Design review of the part built by this model. Coordinates are the model's own, in mm. A direction names the side the tool comes from. Round coordinates to 2 decimals unless told otherwise and drop trailing zeros. Order: outer loops, then holes, each group sorted by start corner. A loop starts at its lowest first (then second) coordinate and runs counter-clockwise, first axis right, second up.
from build123d import *

# Parameters (mm, degrees)
F0_R     = 5.55625
F1_DEPTH = 4.7625
F2_R     = 2.2225
F3_DEPTH = 12.7
F4_R     = 1.5875
F5_DEPTH = 11.5443


# Not quite as in the source:
# - a length typed as a fraction of an inch, garbled in the dataset ("3 / 203.2 mm" for 3/8 in), is restored


with BuildPart() as f1:
    # F0 (on Top) → F1 (new body)
    with BuildSketch(Plane.XY):
        Circle(F0_R)
    extrude(amount=F1_DEPTH)

    # F2 (on face) → F3 (join)
    with BuildSketch(Plane.XY.offset(4.7625)):
        Circle(F2_R)
    extrude(amount=F3_DEPTH)

    # F4 (on face) → F5 (join)
    with BuildSketch(Plane(origin=(0, 0, 0), x_dir=(1, 0, 0), z_dir=(0, 0, -1))):
        Circle(F4_R)
    extrude(amount=F5_DEPTH)


solid = f1.part
1) Take a section at C-C on z = 13.25. Give the boundary of the cut face in (x, y) (1 decimal).
Results:
outline: circle Ø4.4 at (0, 0)
2) For faces 1 (the face through (-0.1, -2.4, 4.762)), 2 (the face through (5.3, 1.67, 2.35)), 3 (the face through (-1.3, -1.2, 0)), list the 3-axis set-ups (+Z, -Z, +X, -X, +Y, -Y) from which the entire face can be reached by the end or side of a thin tool; tool diameter is ignored.
Results:
face 1: +Z
face 2: +Z, -Z
face 3: -Z
3) Take a section at A-A on x = 0. Give the boundary of the cut face in (y, z), plus the area to 3 significant figures.
Results:
outline: (-5.56, 0) - (-1.59, 0) - (-1.59, -11.54) - (1.59, -11.54) - (1.59, 0) - (5.56, 0) - (5.56, 4.76) - (2.22, 4.76) - (2.22, 17.46) - (-2.22, 17.46) - (-2.22, 4.76) - (-5.56, 4.76) - close
area: 146 mm2
4) Take a section at D-D on x = 2.5. Give the boundary of the cut face in (y, z).
Results:
outline: (-4.96, 0) - (4.96, 0) - (4.96, 4.76) - (-4.96, 4.76) - close
5) Clearance check with flat-ended pins moving along their axes: P1, Ø4, axis at y = -0.5, z = -4.5, coming from the -X side; P2, Ø5, axis at x = 1.5, z = 10, coming from the +Y side; P3, Ø6, axis at x = -3, z = -4, coming from the +Y side. State where each tip first meets the part, or that it passes through.
Results:
P1: stops at x = -1.59
P2: stops at y = 2.22
P3: stops at y = 1.59
6) To check wall thickness, follow line 1 along Z through (x, y) = (-3, 3); line 2 along Z through (x, y) = (0.25, -1.75); line 3 along X through (y, z) = (0.25, -9.5). State the ranges of each line that lie inside material, in increasing order.
Results:
line 1: z = 0 to 4.76
line 2: z = 0 to 17.46
line 3: x = -1.57 to 1.57
